Verification items for the finished model (mm, model axes). Face numbers are marked on the shaded views. A direction names the side the tool comes from. Coordinates: 2 decimals unless noted, no trailing zeros. Write each loop counter-clockwise with the first axis right and the second up, starting at its lowest first coordinate (ties: lowest second). Pieces come first, ordered by that corner, then holes. Notation, with made-up numbers: M -27,-16 L -18,-16 A33 cw -18,12 Z; hole C 41.25,-34.5 d1. An arc over 180 degrees is marked long. Answer in a Markdown table with one row per item.
Autodesk Inventor part; units mm, degrees
ref_plane "YZ Plane" through (0, 0, 0) normal (1, 0, 0) x (0, 1, 0)
ref_plane "XZ Plane" through (0, 0, 0) normal (0, 1, 0) x (-1, 0, 0)
ref_plane "XY Plane" through (0, 0, 0) normal (0, 0, 1) x (1, 0, 0)
sketch "Sketch1" plane through (0, 0, 0) normal (0, 1, 0) x (-1, 0, 0)
  line L0 (20, -20) -> (-20, -20)
  line L1 (-20, -20) -> (-20, 20)
  line L2 (-20, 20) -> (20, 20)
  line L3 (20, 20) -> (20, -20)
  line L4 (20, -20) -> (-20, 20) construction
  line L5 (-20, -20) -> (20, 20) construction
  point P0 (0, 0)
  dimension "d0" = 40
  dimension "d1" = 40
extrude "Extrusion1" add sketch "Sketch1" along normal blind 10
sketch "Sketch2" plane through (0, 10, 0) normal (0, 1, 0) x (1, 0, 0)
  line L0 (20, 20) -> (-20, 20)
  line L1 (-20, -20) -> (20, -20)
  line L2 (-20, 20) -> (20, -20)
  circle A0 centre (0, 0) radius 2.5
  dimension "d4" = 5
extrude "Extrusion2" add sketch "Sketch2" along normal blind 10
properties part number "Base"
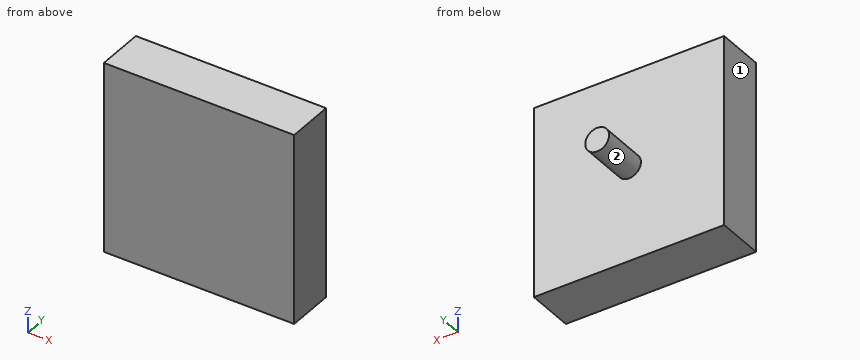
1) Tool access check on the marked faces 1 and 2. Record the directions out of +Z, -Z, +X, -X, +Y, -Y that give a thin tool (end or side, any length) a straight path to the whole face; none if there is none.
Response values:
| item | result |
|---|---|
| face 1 | +Z, -Z, -X, +Y, -Y |
| face 2 | +Y |
2) Thickness scan on L1, parallel to Y at x = -3.5, z = 3.5; L2, parallel to Z at x = 1, y = 17. Record the ranges inside material, lowest first. Write a range as [from, to].
Response values:
| item | result |
|---|---|
| L1 | y = [0, 10] |
| L2 | z = [-2.29, 2.29] |
3) Sectioned sample at C-C (y = 10.75). Record the cut outline in (x, z).
Response values:
| item | result |
|---|---|
| outline | C 0,0 d5 |
4) Sectioned sample at A-A (z = 0). Record the cut outline in (x, y).
Response values:
| item | result |
|---|---|
| outline | M -20,0 L 20,0 L 20,10 L 2.5,10 L 2.5,20 L -2.5,20 L -2.5,10 L -20,10 Z |
5) Sectioned sample at D-D (z = -13.5). Record the cut outline in (x, y), then the cut area to 3 significant figures.
Response values:
| item | result |
|---|---|
| outline | M -20,0 L 20,0 L 20,10 L -20,10 Z |
| area | 400 mm² |
6) Depth check by flat-ended pin: pin 1 (2 mm diameter, centred on x = -5, z = -9.5, fed in from +Y); pin 2 (10 mm diameter, centred on x = 1.5, y = 16, fed in from +Z). Enter the tip coordinate at first touch or a pass-through.
Response values:
| item | result |
|---|---|
| pin 1 | stops at y = 10 |
| pin 2 | stops at z = 2.5 |
7) Sectioned sample at B-B (x = 0). Record the cut outline in (y, z).
Response values:
| item | result |
|---|---|
| outline | M 0,-20 L 10,-20 L 10,-2.5 L 20,-2.5 L 20,2.5 L 10,2.5 L 10,20 L 0,20 Z |
